Verification items for the finished model (mm, model axes). A direction names the side the tool comes from. Give positions to 0.01 mm unless a question says otherwise; leave off trailing zeros. Loops run counter-clockwise (first coordinate to the right, second up) from the corner with the lowest first, then second, coordinate; pieces in that order, holes last. Notation, with made-up numbers: (77.25, -22.75) - (81.25, -22.75) arc R29 cw to (81.25, 4.25) - close; hole circle Ø3 at (-31, -30.75). An arc over 180 degrees is marked (long way). Use one line per item in the form item = value.
```python
from build123d import *

# Parameters (mm, degrees)
ESQUISSE1_W             = 200
ESQUISSE1_H             = 50
BOSS_EXTRU_1_DEPTH      = 20
ESQUISSE2_W             = 20
ESQUISSE2_H             = 20
BOSS_EXTRU_2_DEPTH      = 20
ESQUISSE3_R             = 7.5
ENL_V_MAT_EXTRU_1_DEPTH = 20
ESQUISSE8_R             = 16.25
ENL_V_MAT_EXTRU_3_DEPTH = 12


with BuildPart() as part:
    # Esquisse1 → Boss.-Extru.1 (new body)
    with BuildSketch(Plane.XY):
        Rectangle(ESQUISSE1_W, ESQUISSE1_H)
    extrude(amount=BOSS_EXTRU_1_DEPTH)

    # Esquisse2 → Boss.-Extru.2 (add)
    with BuildSketch(Plane.XY.offset(20)):
        with Locations((-75, 0)):
            Rectangle(ESQUISSE2_W, ESQUISSE2_H)
    extrude(amount=BOSS_EXTRU_2_DEPTH)

    # Esquisse3 → Enlèv. mat.-Extru.1 (cut)
    with BuildSketch(Plane.XY.offset(20)):
        with Locations((75, 0)):
            Circle(ESQUISSE3_R)
    extrude(amount=-ENL_V_MAT_EXTRU_1_DEPTH, mode=Mode.SUBTRACT)

    # Esquisse8 → Enlèv. mat.-Extru.3 (cut)
    with BuildSketch(Plane(origin=(0, 0, 0), x_dir=(-1, 0, 0), z_dir=(0, 0, -1))):
        with Locations((-75, 0)):
            Circle(ESQUISSE8_R)
    extrude(amount=-ENL_V_MAT_EXTRU_3_DEPTH, mode=Mode.SUBTRACT)


solid = part.part
```
1. Depth check by flat-ended pin: pin 1 Ø1.5 at (y, z) = (11.5, 23) entering from +X; pin 2 Ø22 at (x, z) = (-73.5, 32.5) entering from +Y; pin 3 Ø10 at (y, z) = (3.5, 25.5) entering from -X; pin 4 Ø16 at (x, y) = (80.5, 1.5) entering from -Z. Enter the tip coordinate at first touch or a pass-through.
Result set:
pin_1 = through
pin_2 = 10
pin_3 = -85
pin_4 = 12
2. Draft check along X on faces 1 (the flat face through (-1, 0, 0)), 2 (the flat face through (-65, 0, 30)), 3 (the flat face through (68, -3.4, 12)), 4 (the cylindrical face through (91.234, 0.714, 5.916)). Enter one of: released by +X, released by -X, zero draft, split by the parting line, or undercut.
Result set:
face_1 = zero draft
face_2 = released by +X
face_3 = undercut
face_4 = undercut
3. Section check D-D, the plane z = 35. Record the cut outline in (x, y).
Result set:
outline = (-85, -10) - (-65, -10) - (-65, 10) - (-85, 10) - close
4. Section check C-C, the plane z = 15. Record the cut outline in (x, y), then the cut area to 3 significant figures.
Result set:
outline = (-100, -25) - (100, -25) - (100, 25) - (-100, 25) - close; hole circle Ø15 at (75, 0)
area = 9,820 mm²
5. Section check B-B, the plane x = 75. Record the cut outline in (y, z), then the cut area to 3 significant figures.
Result set:
outline = (-25, 0) - (-16.25, 0) - (-16.25, 12) - (-7.5, 12) - (-7.5, 20) - (-25, 20) - close; (7.5, 12) - (16.25, 12) - (16.25, 0) - (25, 0) - (25, 20) - (7.5, 20) - close
area = 490 mm²
6. Tool access check on faces 5 (the flat face through (-75, -10, 30)), 6 (the flat face through (-85, 0, 30)), 7 (the flat face through (-75, 10, 30)), 8 (the flat face through (-75, 0, 40)). Record the directions out of +Z, -Z, +X, -X, +Y, -Y that give a thin tool (end or side, any length) a straight path to the whole face; none if there is none.
Result set:
face_5 = +Z, +X, -X, -Y
face_6 = +Z, -X, +Y, -Y
face_7 = +Z, +X, -X, +Y
face_8 = +Z, +X, -X, +Y, -Y
7. Scan lines: probe 1 along Y at (x, z) = (75, 3); probe 2 along Y at (x, z) = (75, 18); probe 3 along Z at (x, y) = (-25.5, 22). Record each from-to range of solid material in increasing order.
Result set:
probe_1 = -25 to -16.25, 16.25 to 25
probe_2 = -25 to -7.5, 7.5 to 25
probe_3 = 0 to 20
8. Section check A-A, the plane y = 0. Record the cut outline in (x, z), then the cut area to 3 significant figures.
Result set:
outline = (-100, 0) - (58.75, 0) - (58.75, 12) - (67.5, 12) - (67.5, 20) - (-65, 20) - (-65, 40) - (-85, 40) - (-85, 20) - (-100, 20) - close; (82.5, 12) - (91.25, 12) - (91.25, 0) - (100, 0) - (100, 20) - (82.5, 20) - close
area = 3,890 mm²
